Autodesk Inventor part; units mm, degrees
ref_plane "YZ Plane" through (0, 0, 0) normal (1, 0, 0) x (0, 1, 0)
ref_plane "XZ Plane" through (0, 0, 0) normal (0, 1, 0) x (-1, 0, 0)
ref_plane "XY Plane" through (0, 0, 0) normal (0, 0, 1) x (1, 0, 0)
sketch "Sketch1" plane through (0, 0, 0) normal (0, 0, 1) x (1, 0, 0)
  line L0 (-10, -10) -> (10, 10) construction
  line L1 (10, -10) -> (-10, 10) construction
  arc A0 (-10, -9.5) -> (-9.5, -10) centre (-9.5, -9.5) ccw
  arc A1 (-9.5, 10) -> (-10, 9.5) centre (-9.5, 9.5) ccw
  arc A2 (10, 9.5) -> (9.5, 10) centre (9.5, 9.5) ccw
  arc A3 (9.5, -10) -> (10, -9.5) centre (9.5, -9.5) ccw
  line L2 (7, -7) -> (-7, -7) construction
  line L3 (-7, -7) -> (-7, 7) construction
  line L4 (-7, 7) -> (7, 7) construction
  line L5 (7, 7) -> (7, -7) construction
  line L6 (7, -7) -> (-7, 7) construction
  line L7 (-7, -7) -> (7, 7) construction
  circle A4 centre (-7, -7) radius 2
  circle A5 centre (-7, 7) radius 2
  circle A6 centre (7, 7) radius 2
  circle A7 centre (7, -7) radius 2
  circle A8 centre (0, 0) radius 2.15
  line L8 (-8.5, 4.15) -> (-5.1906, 4.15)
  arc A9 (-5.1906, -4.15) -> (-5.1906, 4.15) centre (-8.8, 0) ccw
  line L9 (-5.1906, -4.15) -> (-8.5, -4.15)
  line L10 (-8.5, -4.15) -> (-8.5, -2.7559)
  line L11 (-8.5, 2.5441) -> (-8.5, 4.15)
  line L12 (-5.1906, -4.15) -> (-5.1906, 4.15) construction
  line L13 (-8.5, -2.7559) -> (-10, -2.7559)
  line L14 (-8.5, 2.5441) -> (-10, 2.5441)
  line L15 (-10, 9.5) -> (-10, 2.5441)
  line L16 (-10, -2.7559) -> (-10, -9.5)
  line L17 (4.15, -8.5) -> (2.7559, -8.5)
  line L18 (2.7559, -8.5) -> (2.7559, -10)
  line L19 (4.15, -5.1906) -> (-4.15, -5.1906) construction
  arc A10 (4.15, -5.1906) -> (-4.15, -5.1906) centre (0, -8.8) ccw
  line L20 (7, -7) -> (-7, 7) construction
  line L21 (10, -10) -> (-10, 10) construction
  line L22 (-4.15, -8.5) -> (-4.15, -5.1906)
  line L23 (4.15, -5.1906) -> (4.15, -8.5)
  line L24 (-2.5441, -8.5) -> (-2.5441, -10)
  line L25 (-2.5441, -8.5) -> (-4.15, -8.5)
  line L26 (8.5, 4.15) -> (8.5, 2.7559)
  line L27 (8.5, 2.7559) -> (10, 2.7559)
  line L28 (5.1906, 4.15) -> (5.1906, -4.15) construction
  arc A11 (5.1906, 4.15) -> (5.1906, -4.15) centre (8.8, 0) ccw
  line L29 (7, 7) -> (-7, -7) construction
  line L30 (10, 10) -> (-10, -10) construction
  line L31 (8.5, -4.15) -> (5.1906, -4.15)
  line L32 (5.1906, 4.15) -> (8.5, 4.15)
  line L33 (8.5, -2.5441) -> (10, -2.5441)
  line L34 (8.5, -2.5441) -> (8.5, -4.15)
  line L35 (-4.15, 8.5) -> (-2.7559, 8.5)
  line L36 (-2.7559, 8.5) -> (-2.7559, 10)
  line L37 (-4.15, 5.1906) -> (4.15, 5.1906) construction
  arc A12 (-4.15, 5.1906) -> (4.15, 5.1906) centre (0, 8.8) ccw
  line L38 (-7, 7) -> (7, -7) construction
  line L39 (-10, 10) -> (10, -10) construction
  line L40 (4.15, 8.5) -> (4.15, 5.1906)
  line L41 (-4.15, 5.1906) -> (-4.15, 8.5)
  line L42 (2.5441, 8.5) -> (2.5441, 10)
  line L43 (2.5441, 8.5) -> (4.15, 8.5)
  line L44 (-9.5, -10) -> (-2.5441, -10)
  line L45 (2.7559, -10) -> (9.5, -10)
  line L46 (9.5, 10) -> (2.5441, 10)
  line L47 (-2.7559, 10) -> (-9.5, 10)
  line L48 (10, -9.5) -> (10, -2.5441)
  line L49 (10, 2.7559) -> (10, 9.5)
  line L50 (2292.4151, 1187.1915) -> (2314.8128, 1187.1915)
  circle A13 centre (2303.6139, 1187.1915) radius 2.15
  line L51 (2307.7639, 1192.1343) -> (2307.7639, 1195.3915)
  arc A14 (2307.7639, 1195.3915) -> (2307.4639, 1195.6915) centre (2307.4639, 1195.3915) ccw
  line L52 (2307.4639, 1195.6915) -> (2306.5639, 1195.6915)
  arc A15 (2306.2639, 1195.9915) -> (2306.5639, 1195.6915) centre (2306.5639, 1195.9915) ccw
  line L53 (2306.2639, 1195.9915) -> (2306.2639, 1196.8915)
  arc A16 (2306.5639, 1197.1915) -> (2306.2639, 1196.8915) centre (2306.5639, 1196.8915) ccw
  line L54 (2306.5639, 1197.1915) -> (2313.3139, 1197.1915)
  arc A17 (2313.6139, 1196.8915) -> (2313.3139, 1197.1915) centre (2313.3139, 1196.8915) ccw
  line L55 (2313.6139, 1196.8915) -> (2313.6139, 1190.1415)
  arc A18 (2313.3139, 1189.8415) -> (2313.6139, 1190.1415) centre (2313.3139, 1190.1415) ccw
  line L56 (2313.3139, 1189.8415) -> (2312.4139, 1189.8415)
  arc A19 (2312.1139, 1190.1415) -> (2312.4139, 1189.8415) centre (2312.4139, 1190.1415) ccw
  line L57 (2312.1139, 1190.1415) -> (2312.1139, 1191.0415)
  arc A20 (2312.1139, 1191.0415) -> (2311.8139, 1191.3415) centre (2311.8139, 1191.0415) ccw
  line L58 (2311.8139, 1191.3415) -> (2308.5567, 1191.3415)
  arc A21 (2308.5567, 1191.3415) -> (2308.3217, 1191.2281) centre (2308.5567, 1191.0415) ccw
  arc A22 (2308.3217, 1191.2281) -> (2306.9212, 1187.4988) centre (2313.4048, 1187.1915) ccw
  line L59 (2306.9212, 1187.4988) -> (2306.6139, 1187.1915)
  line L60 (2306.6139, 1187.1915) -> (2306.9212, 1186.8843)
  arc A23 (2306.9212, 1186.8843) -> (2308.3217, 1183.155) centre (2313.4048, 1187.1915) ccw
  arc A24 (2308.3217, 1183.155) -> (2308.5567, 1183.0415) centre (2308.5567, 1183.3415) ccw
  line L61 (2308.5567, 1183.0415) -> (2311.8139, 1183.0415)
  arc A25 (2311.8139, 1183.0415) -> (2312.1139, 1183.3415) centre (2311.8139, 1183.3415) ccw
  line L62 (2312.1139, 1183.3415) -> (2312.1139, 1184.2415)
  arc A26 (2312.4139, 1184.5415) -> (2312.1139, 1184.2415) centre (2312.4139, 1184.2415) ccw
  line L63 (2312.4139, 1184.5415) -> (2313.3139, 1184.5415)
  arc A27 (2313.6139, 1184.2415) -> (2313.3139, 1184.5415) centre (2313.3139, 1184.2415) ccw
  line L64 (2313.6139, 1184.2415) -> (2313.6139, 1177.4915)
  arc A28 (2313.3139, 1177.1915) -> (2313.6139, 1177.4915) centre (2313.3139, 1177.4915) ccw
  line L65 (2313.3139, 1177.1915) -> (2306.5639, 1177.1915)
  arc A29 (2306.2639, 1177.4915) -> (2306.5639, 1177.1915) centre (2306.5639, 1177.4915) ccw
  line L66 (2306.2639, 1177.4915) -> (2306.2639, 1178.3915)
  arc A30 (2306.5639, 1178.6915) -> (2306.2639, 1178.3915) centre (2306.5639, 1178.3915) ccw
  line L67 (2306.5639, 1178.6915) -> (2307.4639, 1178.6915)
  arc A31 (2307.4639, 1178.6915) -> (2307.7639, 1178.9915) centre (2307.4639, 1178.9915) ccw
  line L68 (2307.7639, 1178.9915) -> (2307.7639, 1182.2488)
  arc A32 (2307.7639, 1182.2488) -> (2307.6505, 1182.4837) centre (2307.4639, 1182.2488) ccw
  arc A33 (2307.6505, 1182.4837) -> (2303.9212, 1183.8843) centre (2303.6139, 1177.4007) ccw
  line L69 (2303.9212, 1183.8843) -> (2303.6139, 1184.1915)
  line L70 (2303.6139, 1184.1915) -> (2303.3066, 1183.8843)
  arc A34 (2303.3066, 1183.8843) -> (2299.5774, 1182.4837) centre (2303.6139, 1177.4007) ccw
  arc A35 (2299.5774, 1182.4837) -> (2299.4639, 1182.2488) centre (2299.7639, 1182.2488) ccw
  line L71 (2299.4639, 1182.2488) -> (2299.4639, 1178.9915)
  arc A36 (2299.4639, 1178.9915) -> (2299.7639, 1178.6915) centre (2299.7639, 1178.9915) ccw
  line L72 (2299.7639, 1178.6915) -> (2300.6639, 1178.6915)
  arc A37 (2300.9639, 1178.3915) -> (2300.6639, 1178.6915) centre (2300.6639, 1178.3915) ccw
  line L73 (2300.9639, 1178.3915) -> (2300.9639, 1177.4915)
  arc A38 (2300.6639, 1177.1915) -> (2300.9639, 1177.4915) centre (2300.6639, 1177.4915) ccw
  line L74 (2300.6639, 1177.1915) -> (2293.9139, 1177.1915)
  arc A39 (2293.6139, 1177.4915) -> (2293.9139, 1177.1915) centre (2293.9139, 1177.4915) ccw
  line L75 (2293.6139, 1177.4915) -> (2293.6139, 1184.2415)
  arc A40 (2293.9139, 1184.5415) -> (2293.6139, 1184.2415) centre (2293.9139, 1184.2415) ccw
  line L76 (2293.9139, 1184.5415) -> (2294.8139, 1184.5415)
  arc A41 (2295.1139, 1184.2415) -> (2294.8139, 1184.5415) centre (2294.8139, 1184.2415) ccw
  line L77 (2295.1139, 1184.2415) -> (2295.1139, 1183.3415)
  arc A42 (2295.1139, 1183.3415) -> (2295.4139, 1183.0415) centre (2295.4139, 1183.3415) ccw
  line L78 (2295.4139, 1183.0415) -> (2298.6712, 1183.0415)
  arc A43 (2298.6712, 1183.0415) -> (2298.9061, 1183.155) centre (2298.6712, 1183.3415) ccw
  arc A44 (2298.9061, 1183.155) -> (2300.3066, 1186.8843) centre (2293.8231, 1187.1915) ccw
  line L79 (2300.3066, 1186.8843) -> (2300.6139, 1187.1915)
  line L80 (2300.6139, 1187.1915) -> (2300.3066, 1187.4988)
  arc A45 (2300.3066, 1187.4988) -> (2298.9061, 1191.2281) centre (2293.8231, 1187.1915) ccw
  arc A46 (2298.9061, 1191.2281) -> (2298.6712, 1191.3415) centre (2298.6712, 1191.0415) ccw
  line L81 (2298.6712, 1191.3415) -> (2295.4139, 1191.3415)
  arc A47 (2295.4139, 1191.3415) -> (2295.1139, 1191.0415) centre (2295.4139, 1191.0415) ccw
  line L82 (2295.1139, 1191.0415) -> (2295.1139, 1190.1415)
  arc A48 (2294.8139, 1189.8415) -> (2295.1139, 1190.1415) centre (2294.8139, 1190.1415) ccw
  line L83 (2294.8139, 1189.8415) -> (2293.9139, 1189.8415)
  arc A49 (2293.6139, 1190.1415) -> (2293.9139, 1189.8415) centre (2293.9139, 1190.1415) ccw
  line L84 (2293.6139, 1190.1415) -> (2293.6139, 1196.8915)
  arc A50 (2293.9139, 1197.1915) -> (2293.6139, 1196.8915) centre (2293.9139, 1196.8915) ccw
  line L85 (2293.9139, 1197.1915) -> (2300.6639, 1197.1915)
  arc A51 (2300.9639, 1196.8915) -> (2300.6639, 1197.1915) centre (2300.6639, 1196.8915) ccw
  line L86 (2300.9639, 1196.8915) -> (2300.9639, 1195.9915)
  arc A52 (2300.6639, 1195.6915) -> (2300.9639, 1195.9915) centre (2300.6639, 1195.9915) ccw
  line L87 (2300.6639, 1195.6915) -> (2299.7639, 1195.6915)
  arc A53 (2299.7639, 1195.6915) -> (2299.4639, 1195.3915) centre (2299.7639, 1195.3915) ccw
  line L88 (2299.4639, 1195.3915) -> (2299.4639, 1192.1343)
  arc A54 (2299.4639, 1192.1343) -> (2299.5774, 1191.8994) centre (2299.7639, 1192.1343) ccw
  arc A55 (2299.5774, 1191.8994) -> (2303.3066, 1190.4988) centre (2303.6139, 1196.9824) ccw
  line L89 (2303.3066, 1190.4988) -> (2303.6139, 1190.1915)
  line L90 (2303.6139, 1190.1915) -> (2303.9212, 1190.4988)
  arc A56 (2303.9212, 1190.4988) -> (2307.6505, 1191.8994) centre (2303.6139, 1196.9824) ccw
  arc A57 (2307.6505, 1191.8994) -> (2307.7639, 1192.1343) centre (2307.4639, 1192.1343) ccw
  line L91 (2294.1139, 1194.1915) -> (2299.1139, 1194.1915)
  line L92 (2296.6139, 1196.6915) -> (2296.6139, 1191.6915)
  circle A58 centre (2296.6139, 1194.1915) radius 2
  line L93 (2294.1139, 1180.1915) -> (2299.1139, 1180.1915)
  line L94 (2296.6139, 1177.6915) -> (2296.6139, 1182.6915)
  circle A59 centre (2296.6139, 1180.1915) radius 2
  line L95 (2303.6139, 1198.3904) -> (2303.6139, 1175.9927)
  line L96 (2313.1139, 1194.1915) -> (2308.1139, 1194.1915)
  line L97 (2310.6139, 1196.6915) -> (2310.6139, 1191.6915)
  circle A60 centre (2310.6139, 1194.1915) radius 2
  circle A61 centre (2310.6139, 1180.1915) radius 2
  line L98 (2310.6139, 1177.6915) -> (2310.6139, 1182.6915)
  line L99 (2313.1139, 1180.1915) -> (2308.1139, 1180.1915)
  point P0 (-10, 0)
  point P1 (-5.8595, 0)
  point P2 (-5.1906, 0)
  point P3 (-10, 0)
  point P4 (0, -5.8595)
  point P5 (0, -5.1906)
  point P6 (5.8595, 0)
  point P7 (5.1906, 0)
  point P8 (0, 5.8595)
  point P9 (0, 5.1906)
  dimension "d0" = 20
  dimension "d1" = 20
  dimension "d2" = 0.5
  dimension "d3" = 14
  dimension "d4" = 14
  dimension "d5" = 4
  dimension "d6" = 4.3
  dimension "d13" = 5.5
  dimension "d14" = 8.3
  dimension "d16" = 5.3
  dimension "d17" = 6.7
  dimension "d18" = 1.5
  dimension "d21" = 360
extrude "Extrusion1" add sketch "Sketch1" along normal blind 176 contours L16 L13 L10 L9 A9 L8 L11 L14 L15 A1 L47 L36 L35 L41 A12 L40 L43 L42 L46 A2 L49 L27 L26 L32 A11 L31 L34 L33 L48 A3 L45 L18 L17 L23 A10 L22 L25 L24 L44 A0
properties part number "Profile"
The model under review builds one solid part; all positions refer to its coordinate system, in mm. A direction names the side the tool comes from. Give positions to 0.01 mm unless a question says otherwise; leave off trailing zeros. Write each loop counter-clockwise with the first axis right and the second up, starting at its lowest first coordinate (ties: lowest second). Pieces come first, ordered by that corner, then holes. Notation, with made-up numbers: (17, 1) -> (60, 1) arc R26 ccw to (60, 31) -> close; hole circle Ø1 at (4, -31.75). An arc over 180 degrees is marked (long way). Put each result on its own line as item: value.
(1) The part is to be moulded in two halves that separate along Y. For faces 3 (the flat face through (-10, 6, 87)), 4 (the flat face through (-6, -10, 87)), 5 (the cylindrical face through (-9, 7, 87)), say which applies: pulls with the +Y half, pulls with the -Y half, needs draft (parallel to the pull), parting line crosses it, or undercut.
Results are:
face 3: needs draft
face 4: pulls with the -Y half
face 5: undercut
(2) For pin 1 Ø2 at (y, z) = (1, 22) entering from -X, flat-tipped, find the tip position at first contact; note if it passes through.
Results are:
pin 1: x = -3.68
(3) We need section A-A, the plane y = -7. Give the boundary of the cut face in (x, z).
Results are:
outline: (-10, 0) -> (-9, 0) -> (-9, 176) -> (-10, 176) -> close; (-5, 0) -> (-4.15, 0) -> (-4.15, 176) -> (-5, 176) -> close; (4.15, 0) -> (5, 0) -> (5, 176) -> (4.15, 176) -> close; (9, 0) -> (10, 0) -> (10, 176) -> (9, 176) -> close
(4) Tool access review of faces 1 (the flat face through (-6, 10, 87)), 2 (the cylindrical face through (0.1, 3.3, 86.8)): name each direction out of +Z, -Z, +X, -X, +Y, -Y from which nothing blocks a thin tool from reaching the whole face with its end or side.
Results are:
face 1: +Z, -Z, +X, -X, +Y
face 2: +Z, -Z
(5) We need section D-D, the plane z = 154. State how many separate pieces and enclosed holes the cut face has, and give its area (3 significant figures).
Results are:
separate pieces: 1
enclosed holes: 5
area: 150 mm²
(6) To check wall thickness, follow probe 1 along Y at (x, z) = (-7, 129); probe 2 along Y at (x, z) = (4, 55.5); probe 3 along Y at (x, z) = (0, 56). State the ranges of each line that lie inside material, in increasing order. Write a range as from..to.
Results are:
probe 1: -10..-9, -5..-4.15, 4.15..5, 9..10
probe 2: -10..-8.5, -5.03..-2.69, 2.69..5.03, 8.5..10
probe 3: -3.3..-2.15, 2.15..3.3
(7) We need section B-B, the plane y = 0. Give the boundary of the cut face in (x, z).
Results are:
outline: (-3.3, 0) -> (-2.15, 0) -> (-2.15, 176) -> (-3.3, 176) -> close; (2.15, 0) -> (3.3, 0) -> (3.3, 176) -> (2.15, 176) -> close
